Read the model definition and answer for the solid it produces. Units are mm, in the model's axes. A direction names the side the tool comes from. Coordinates: 2 decimals unless noted, no trailing zeros. Loops run counter-clockwise (first coordinate to the right, second up) from the corner with the lowest first, then second, coordinate; pieces in that order, holes last. Notation, with made-up numbers: (73.25, -39.75) -> (99.25, -39.75) arc R18 cw to (99.25, -35.75) -> close; hole circle Ø1 at (22.5, 74.25). An arc over 180 degrees is marked (long way). Answer as a JSON object with one key per item and string values. Group by question number.
Q1. The part is cut by section A-A on z = 0. Write down the section's boundary in (x, y) (3 decimals).
Q2. Determine the mould class of faces 5 (the cylindrical face through (-5.66, 3.07, 1.5)), 6 (the flat face through (2, 0, 2)), 7 (the flat face through (3, 6.54, 0)) for opening direction Y: released by +Y, released by -Y, zero draft, split by the parting line, or undercut.
Q3. For faces 1 (the cylindrical face through (1.5, 3.07, 5.66)), 2 (the cylindrical face through (-6.516, 21.245, -1.386)), 3 (the cylindrical face through (3.853, 15.808, -1.214)), 4 (the flat face through (4, 24.82, 2)), determine the directions among +Z, -Z, +X, -X, +Y, -Y from which every point of the face is accessible in a straight line to the end or side of a thin tool.
Q4. Each of these flat-tipped pins is pushed along its axis until it touches: P1, Ø1, axis at y = 18, z = -2, coming from the +X side; P2, Ø2.5, axis at y = 3, z = 0, coming from the -X side; P3, Ø2, axis at y = 3.5, z = 5.5, coming from the +X side. Where does it stop, or does it pass through?
Q5. The part is cut by section C-C on y = 13.5. Write down the section's boundary in (x, z), and give its area (3 significant figures).
Q6. The part is cut by section D-D on z = 6.5. State how many separate pieces and enclosed holes the cut face has, and give its area (3 significant figures).
Q7. The part is cut by section B-B on y = 21.82. Write down the section's boundary in (x, z), and give its area (3 significant figures).
Q8. Straight lines are drawn through the part: line 1 along Y through (x, z) = (0, 6.25); line 2 along Z through (x, y) = (0, 17); line 3 along Z through (x, y) = (-1.75, 23). For each, find the intervals that lie inside material, in ascending order. Write a range as [from, to].
from build123d import *

# Parameters (mm, degrees)
SKETCH1_R           = 9.36
BOSS_EXTRUDE1_DEPTH = 24.82
SKETCH2_R           = 2.545
CUT_EXTRUDE1_DEPTH  = 25.82
CUT_EXTRUDE2_START  = 24.82
SKETCH2_3_R         = 4.04
SKETCH2_3_R_2       = 2.545
CUT_EXTRUDE2_DEPTH  = 18.28
CHAMFER1_SIZE       = 0.5
SKETCH3_R           = 1.5
CUT_EXTRUDE3_DEPTH  = 18.28
CIRPATTERN1_COUNT   = 2
CIRPATTERN1_ANGLE   = 90


with BuildPart() as part:
    # Sketch1 → Boss-Extrude1 (new body)
    with BuildSketch(Plane(origin=(0, 0, 0), x_dir=(1, 0, 0), z_dir=(0, 1, 0))):
        Circle(SKETCH1_R)
    extrude(amount=BOSS_EXTRUDE1_DEPTH)

    # Sketch2 → Cut-Extrude1 (cut, through all)
    with BuildSketch(Plane(origin=(0, 0, 0), x_dir=(1, 0, 0), z_dir=(0, 1, 0))):
        Circle(SKETCH2_R)
    extrude(amount=CUT_EXTRUDE1_DEPTH, mode=Mode.SUBTRACT)

    # Sketch2<3> → Cut-Extrude2 (cut)
    with BuildSketch(Plane(origin=(0, 0, 0), x_dir=(1, 0, 0), z_dir=(0, 1, 0)).offset(CUT_EXTRUDE2_START)):
        Circle(SKETCH2_3_R)
        Circle(SKETCH2_3_R_2, mode=Mode.SUBTRACT)
    extrude(amount=-CUT_EXTRUDE2_DEPTH, mode=Mode.SUBTRACT)

    # Chamfer1
    chamfer1_edges = [part.edges().sort_by_distance(p)[0] for p in [
        (-9.36, 0, 0),
        (-9.36, 24.82, 0),
    ]]
    chamfer(chamfer1_edges, length=CHAMFER1_SIZE)

    # Sketch3 → Cut-Extrude3 (cut)
    with BuildSketch(Plane(origin=(0, 0, 0), x_dir=(0, 0, -1), z_dir=(1, 0, 0))):
        with Locations((0, 21.82)):
            Circle(SKETCH3_R)
        with Locations((0, 3)):
            Circle(SKETCH3_R)
    cut_extrude3 = extrude(amount=-CUT_EXTRUDE3_DEPTH, mode=Mode.SUBTRACT)

    # CirPattern1: Cut-Extrude3 ×2 about axis
    cirpattern1_axis = Axis((0, 24.82, 0), (0, 1, 0))
    for i in range(1, CIRPATTERN1_COUNT):
        add(cut_extrude3.rotate(cirpattern1_axis, i * CIRPATTERN1_ANGLE / (CIRPATTERN1_COUNT - 1)), mode=Mode.SUBTRACT)


solid = part.part
Final values:
{
 "1": {"outline": "(-9.36, 0.5) -> (-8.86, 0) -> (-2.545, 0) -> (-2.545, 1.5) -> (-9.36, 1.5) -> close; (-9.36, 4.5) -> (-2.545, 4.5) -> (-2.545, 6.54) -> (-4.04, 6.54) -> (-4.04, 20.32) -> (-9.36, 20.32) -> close; (-9.36, 23.32) -> (-4.04, 23.32) -> (-4.04, 24.82) -> (-8.86, 24.82) -> (-9.36, 24.32) -> close; (2.545, 0) -> (8.86, 0) -> (9.36, 0.5) -> (9.36, 24.32) -> (8.86, 24.82) -> (4.04, 24.82) -> (4.04, 6.54) -> (2.545, 6.54) -> close"},
 "2": {"face 5": "undercut", "face 6": "released by -Y", "face 7": "released by +Y"},
 "3": {"face 1": "+Z", "face 2": "-X", "face 3": "+Y", "face 4": "+Z, -Z, +X, -X, +Y"},
 "4": {"P1": "stops at x = 9.24", "P2": "stops at x = 2.22", "P3": "stops at x = 8.21"},
 "5": {"outline": "circle Ø18.72 at (0, 0); hole circle Ø8.08 at (0, 0)", "area": "224 mm2"},
 "6": {"separate pieces": "1", "enclosed holes": "2", "area": "319 mm2"},
 "7": {"outline": "(-9.24, -1.5) arc R9.36 ccw (long way) to (1.5, 9.24) -> (1.5, 3.75) arc R4.04 cw (long way) to (-3.75, -1.5) -> close; (-9.24, 1.5) -> (-3.75, 1.5) arc R4.04 cw to (-1.5, 3.75) -> (-1.5, 9.24) arc R9.36 ccw to start", "area": "192 mm2"},
 "8": {"line 1": "y = [0, 1.5], [4.5, 20.32], [23.32, 24.82]", "line 2": "z = [-9.36, -4.04], [4.04, 9.36]", "line 3": "z = [-9.19, -3.64], [3.64, 9.19]"}
}
